Design review of the part built by this model. Coordinates are the model's own, in mm. A direction names the side the tool comes from. Coordinates: 2 decimals unless noted, no trailing zeros. Write each loop counter-clockwise with the first axis right and the second up, starting at its lowest first coordinate (ties: lowest second). Pieces come first, ordered by that corner, then holes.
Q1. Take a section at C-C, the plane x = -5. Write out the cut boundary in (y, z), plus the area to 3 significant figures.
Q2. For pin 1 Ø4.5 at (y, z) = (57, -50) entering from -X; pin 2 Ø3 at (x, y) = (-36, 64.5) entering from -Z; pin 3 Ø4 at (x, y) = (-27.5, 21) entering from -Z, all flat-tipped, find the tip position at first contact; note any pin that passes through.
Q3. Take a section at B-B, the plane z = 37. Write out the cut boundary in (x, y), plus the area to 3 significant figures.
Q4. For faces 1 (the cylindrical face through (1.479, -47.804, 47.711)), 2 (the flat face through (0, 55.1, -51.7)), 3 (the flat face through (-21.816, -21.067, -63.028)), list the 3-axis set-ups (+Z, -Z, +X, -X, +Y, -Y) from which the entire face can be reached by the end or side of a thin tool; tool diameter is ignored.
Q5. For L1, parallel to Y at x = -6.5, z = 40; L2, parallel to Y at x = -36.5, z = -45, list the stretches that pass through material, from the lowest coordinate up.
Q6. Take a section at A-A, the plane y = 40.5. Write out the cut boundary in (x, z).
Q7. The part is to be moulded in two halves that separate along X. For faces 4 (the flat face through (-17, 27, -68)), 5 (the flat face through (-17, 15, -68)), 6 (the flat face through (0, -55.3, 51.9)), 7 (the flat face through (-26.071, 17.098, -67.157)), say which applies: released by +X, released by -X, zero draft, split by the parting line, or undercut.
from build123d import *

# Parameters (mm, degrees)
SKETCH2_W           = 142
SKETCH2_H           = 142
SKETCH2_W_2         = 122
SKETCH2_H_2         = 122
BOSS_EXTRUDE1_DEPTH = 3
SKETCH2_4_W         = 142
SKETCH2_4_H         = 142
SKETCH2_4_W_2       = 122
SKETCH2_4_H_2       = 122
BOSS_EXTRUDE2_DEPTH = 30
BOSS_EXTRUDE3_DEPTH = 10
CUT_EXTRUDE5_START  = -132
CUT_EXTRUDE5_DEPTH  = 122
SKETCH15_W          = 122
SKETCH15_H          = 10
BOSS_EXTRUDE4_DEPTH = 10
CAVITY2_START       = -40
CAVITY2_DEPTH       = 10
CAVITY2_START_2     = -61
CAVITY2_2_DEPTH     = 133
CUT_EXTRUDE8_DEPTH  = 25.287407973
CUT_EXTRUDE9_START  = -6
CUT_EXTRUDE9_DEPTH  = 10


with BuildPart() as part:
    # Sketch2 → Boss-Extrude1 (new body)
    # profile 1 of 5: a face of its own
    with BuildSketch(Plane.YZ):
        Rectangle(SKETCH2_W, SKETCH2_H)
        Rectangle(SKETCH2_W_2, SKETCH2_H_2, mode=Mode.SUBTRACT)
    # profile 2 of 5: a face of its own
    with BuildSketch(Plane.YZ):
        with BuildLine():
            Line((-61, 61), (-61, 46))
            Line((-61, 46), (-52, 46))
            ThreePointArc((-52, 46), (-47.757359313, 47.757359313), (-46, 52))
            Line((-46, 52), (-46, 61))
            Line((-46, 61), (-61, 61))
        make_face()
        with BuildLine():
            ThreePointArc((-49.585786438, 52.414213562), (-49.585786438, 49.585786438), (-52.414213562, 49.585786438))
            Line((-52.414213562, 49.585786438), (-55.242640687, 52.414213562))
            ThreePointArc((-55.242640687, 52.414213562), (-55.242640687, 55.242640687), (-52.414213562, 55.242640687))
            Line((-52.414213562, 55.242640687), (-49.585786438, 52.414213562))
        make_face(mode=Mode.SUBTRACT)
    # profile 3 of 5: a face of its own
    with BuildSketch(Plane.YZ):
        with BuildLine():
            Line((52, 46), (61, 46))
            Line((61, 46), (61, 61))
            Line((61, 61), (46, 61))
            Line((46, 61), (46, 52))
            ThreePointArc((46, 52), (47.757359313, 47.757359313), (52, 46))
        make_face()
        with BuildLine():
            ThreePointArc((52.414213562, 49.585786438), (49.585786438, 49.585786438), (49.585786438, 52.414213562))
            Line((49.585786438, 52.414213562), (52.414213562, 55.242640687))
            ThreePointArc((52.414213562, 55.242640687), (55.242640687, 55.242640687), (55.242640687, 52.414213562))
            Line((55.242640687, 52.414213562), (52.414213562, 49.585786438))
        make_face(mode=Mode.SUBTRACT)
    # profile 4 of 5: a face of its own
    with BuildSketch(Plane.YZ):
        with BuildLine():
            Line((46, -52), (46, -61))
            Line((46, -61), (61, -61))
            Line((61, -61), (61, -46))
            Line((61, -46), (52, -46))
            ThreePointArc((52, -46), (47.757359313, -47.757359313), (46, -52))
        make_face()
        with BuildLine():
            ThreePointArc((49.585786438, -52.414213562), (49.585786438, -49.585786438), (52.414213562, -49.585786438))
            Line((52.414213562, -49.585786438), (55.242640687, -52.414213562))
            ThreePointArc((55.242640687, -52.414213562), (55.242640687, -55.242640687), (52.414213562, -55.242640687))
            Line((52.414213562, -55.242640687), (49.585786438, -52.414213562))
        make_face(mode=Mode.SUBTRACT)
    # profile 5 of 5: a face of its own
    with BuildSketch(Plane.YZ):
        with BuildLine():
            Line((-61, -46), (-61, -61))
            Line((-61, -61), (-46, -61))
            Line((-46, -61), (-46, -52))
            ThreePointArc((-46, -52), (-47.757359313, -47.757359313), (-52, -46))
            Line((-52, -46), (-61, -46))
        make_face()
        with BuildLine():
            ThreePointArc((-52.414213562, -49.585786438), (-49.585786438, -49.585786438), (-49.585786438, -52.414213562))
            Line((-49.585786438, -52.414213562), (-52.414213562, -55.242640687))
            ThreePointArc((-52.414213562, -55.242640687), (-55.242640687, -55.242640687), (-55.242640687, -52.414213562))
            Line((-55.242640687, -52.414213562), (-52.414213562, -49.585786438))
        make_face(mode=Mode.SUBTRACT)
    extrude(amount=BOSS_EXTRUDE1_DEPTH)

    # Sketch2<4> → Boss-Extrude2 (add)
    with BuildSketch(Plane.YZ):
        Rectangle(SKETCH2_4_W, SKETCH2_4_H)
        Rectangle(SKETCH2_4_W_2, SKETCH2_4_H_2, mode=Mode.SUBTRACT)
    extrude(amount=-BOSS_EXTRUDE2_DEPTH)

    # Sketch3 → Boss-Extrude3 (add)
    with BuildSketch(Plane(origin=(-30, 0, 0), x_dir=(0, -1, 0), z_dir=(-1, 0, 0))):
        Polygon((-61, -61), (-61, 61), (-61, 71), (-71, 71), (-71, -71), (71, -71), (71, 71), (61, 71), (61, 61), (61, -61), align=None)
    extrude(amount=BOSS_EXTRUDE3_DEPTH)

    # Sketch11 → Cut-Extrude5 (cut)
    with BuildSketch(Plane(origin=(0, 71, 0), x_dir=(-1, 0, 0), z_dir=(0, 1, 0)).offset(CUT_EXTRUDE5_START)):
        Polygon((14.712592027, -65), (19, -65), (24.712592027, -61), (14.712592027, -61), align=None)
    extrude(amount=CUT_EXTRUDE5_DEPTH, mode=Mode.SUBTRACT)

    # Sketch15 → Boss-Extrude4 (add)
    with BuildSketch(Plane(origin=(-30, 0, 0), x_dir=(0, -1, 0), z_dir=(-1, 0, 0))):
        with Locations((0, 66)):
            Rectangle(SKETCH15_W, SKETCH15_H)
    extrude(amount=BOSS_EXTRUDE4_DEPTH)

    # Cavity2: read off the stored shape, not the designer's step
    # Cavity2 outline → Cavity2 (cut)
    with BuildSketch(Plane.YZ.offset(CAVITY2_START)):
        Polygon((19.254896882, -65), (22.745103118, -65), (27, -69.254896882), (24, -71), (71, -71), (71, 71), (67, 71), (67, -61), (-67, -61), (-67, 71), (-71, 71), (-71, -71), (18, -71), (15, -69.254896882), align=None)
    extrude(amount=CAVITY2_DEPTH, mode=Mode.SUBTRACT)

    # Cavity2 2 outline → Cavity2 2 (cut)
    with BuildSketch(Plane.XY.offset(CAVITY2_START_2)):
        Polygon((-30, -67), (-30, -64), (-33, -67), align=None)
        Polygon((-30, 64), (-30, 67), (-33, 67), align=None)
    extrude(amount=CAVITY2_2_DEPTH, mode=Mode.SUBTRACT)

    # Sketch16 → Cut-Extrude8 (cut)
    with BuildSketch(Plane(origin=(-40, 0, 0), x_dir=(0, -1, 0), z_dir=(-1, 0, 0))):
        Polygon((-22.745103118, -65), (-27, -69.254896882), (-24, -71), (-18, -71), (-15, -69.254896882), (-19.254896882, -65), align=None)
    extrude(amount=-CUT_EXTRUDE8_DEPTH, mode=Mode.SUBTRACT)

    # Sketch14 → Cut-Extrude9 (cut)
    with BuildSketch(Plane.XY.offset(-65).offset(CUT_EXTRUDE9_START)):
        Polygon((-19.712592027, 15), (-14.712592027, 15), (-14.712592027, 27), (-19.712592027, 27), (-25.712592027, 21), align=None)
    extrude(amount=CUT_EXTRUDE9_DEPTH, mode=Mode.SUBTRACT)


solid = part.part
Responses:
1. outline: (-71, -71) - (71, -71) - (71, 71) - (-71, 71) - close; hole (-61, -61) - (61, -61) - (61, 61) - (-61, 61) - close
1. area: 5,280 mm2
2. pin 1: stops at x = 0
2. pin 2: stops at z = -61
2. pin 3: stops at z = -65.25
3. outline: (-40, -67) - (-33, -67) - (-30, -64) - (-30, -71) - (3, -71) - (3, -61) - (-40, -61) - close; (-40, 61) - (3, 61) - (3, 71) - (-30, 71) - (-30, 64) - (-33, 67) - (-40, 67) - close
3. area: 771 mm2
4. face 1: +X, -X
4. face 2: -X
4. face 3: none
5. L1: y = -71 to -61, 61 to 71
5. L2: y = -67 to -61, 61 to 67
6. outline: (-40, 61) - (3, 61) - (3, 71) - (-40, 71) - close; (-30, -71) - (3, -71) - (3, -61) - (-14.71, -61) - (-14.71, -65) - (-19, -65) - (-24.71, -61) - (-30, -61) - close
7. face 4: undercut
7. face 5: undercut
7. face 6: released by -X
7. face 7: zero draft
